Verification items for this drawing (mm, ordinates from the low corner). Give positions to 0.01 mm unless a question says otherwise; leave off trailing zeros. Order: outer loops, then holes, each group sorted by start corner. A loop starts at its lowest first (then second) coordinate and runs counter-clockwise, first axis right, second up. Notation, with made-up numbers: M 67,49 L 117,49 A20 cw 117,76 Z; hole C 57.5,8 d3. An arc over 180 degrees is marked long. Return JSON: item names as keys, results as strings. Group by question number.
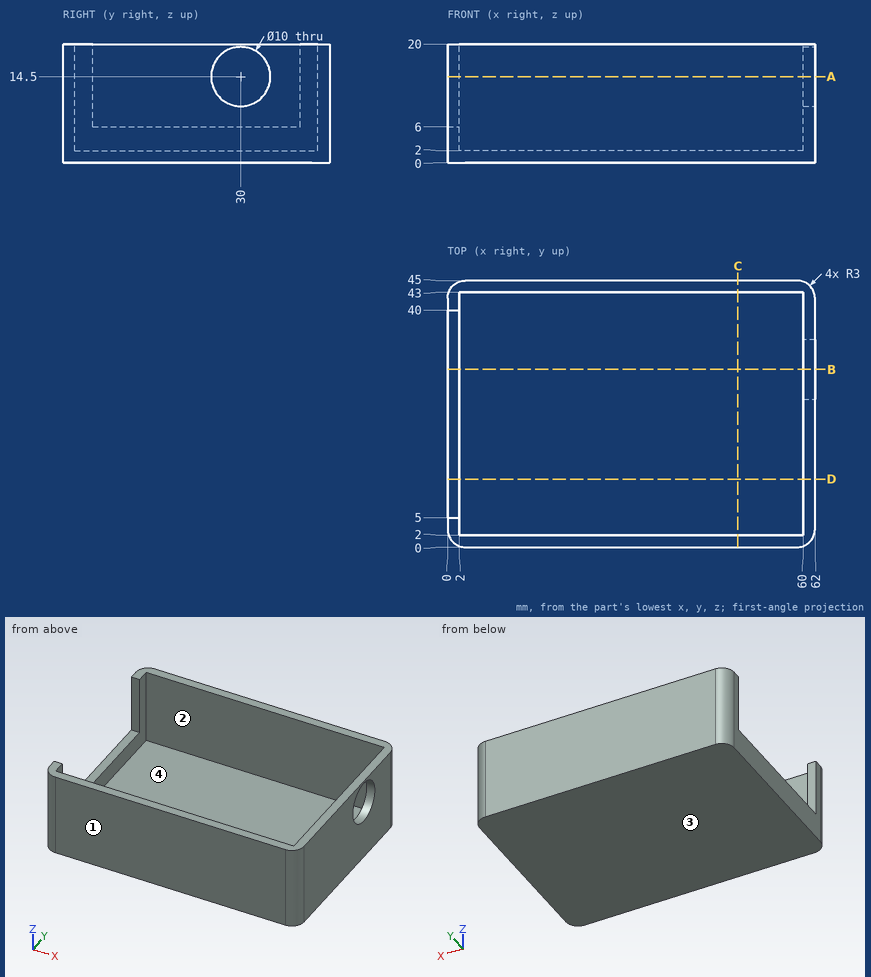
1) Sectioned sample at A-A on z = 14.5. Record the boundary of the cut face in (x, y).
2) Material ranges on line 1 along Y through (x, z) = (30, 13.75); line 2 along X through (y, z) = (29.5, 3.5); line 3 along Z through (x, y) = (61, 30), recorded low to high.
3) Depth check by flat-ended pin: P1, Ø12.5, axis at x = 21, y = 32.5, coming from the +Z side; P2, Ø1, axis at x = 1.5, z = 14.5, coming from the -Y side; P3, Ø1, axis at x = 1, y = 30, coming from the +Z side. Enter the tip coordinate at first touch or a pass-through.
4) Sectioned sample at B-B on y = 30. Record the boundary of the cut face in (x, z), then the cut area to 3 significant figures.
5) Release check for a two-part mould opening along Y. For the marked faces 1, 2, 3 and 4 record: released by +Y, released by -Y, zero draft, split by the parting line, or undercut.
6) Sectioned sample at D-D on y = 11.5. Record the boundary of the cut face in (x, z), then the cut area to 3 significant figures.
7) Sectioned sample at C-C on x = 49. Record the boundary of the cut face in (y, z), then the cut area to 3 significant figures.
Reply:
{
 "1": {"outline": "M 0,3 A3 ccw 3,0 L 59,0 A3 ccw 62,3 L 62,25 L 60,25 L 60,2 L 2,2 L 2,5 L 0,5 Z; M 0,40 L 2,40 L 2,43 L 60,43 L 60,35 L 62,35 L 62,42 A3 ccw 59,45 L 3,45 A3 ccw 0,42 Z"},
 "2": {"line 1": "0 to 2, 43 to 45", "line 2": "0 to 2, 60 to 62", "line 3": "0 to 9.5, 19.5 to 20"},
 "3": {"P1": "z = 2", "P2": "y = 0.17", "P3": "z = 6"},
 "4": {"outline": "M 0,0 L 62,0 L 62,9.5 L 60,9.5 L 60,2 L 2,2 L 2,6 L 0,6 Z; M 60,19.5 L 62,19.5 L 62,20 L 60,20 Z", "area": "148 mm^2"},
 "5": {"face 1": "released by -Y", "face 2": "undercut", "face 3": "zero draft", "face 4": "undercut"},
 "6": {"outline": "M 0,0 L 62,0 L 62,20 L 60,20 L 60,2 L 2,2 L 2,6 L 0,6 Z", "area": "168 mm^2"},
 "7": {"outline": "M 0,0 L 45,0 L 45,20 L 43,20 L 43,2 L 2,2 L 2,20 L 0,20 Z", "area": "162 mm^2"}
}
